The drawing under review shows one solid part. Ordinate dimensions are in mm from its lowest x, y, z. Coordinates: 2 decimals unless noted, no trailing zeros. Loops run counter-clockwise (first coordinate to the right, second up) from the corner with the lowest first, then second, coordinate; pieces in that order, holes last.
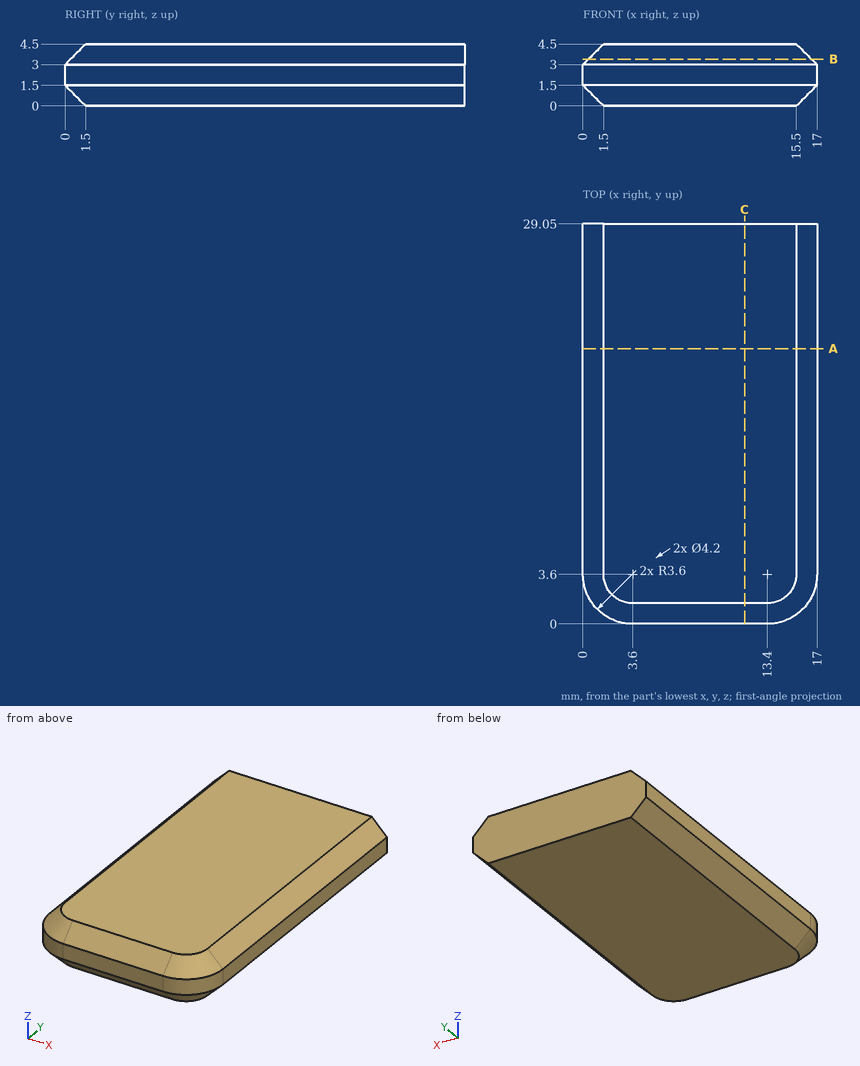
Q1. Take a section at B-B, the plane z = 3.4. Write out the cut boundary in (x, y), then the cut area to 3 significant figures.
Q2. Take a section at A-A, the plane y = 20. Write out the cut boundary in (x, z).
Q3. Take a section at C-C, the plane x = 11.75. Write out the cut boundary in (y, z).
Q4. For line 1 (Y direction, x = 12, z = 0.4); line 2 (Y direction, x = 6.75, z = 0.25); line 3 (Z direction, x = 16.25, y = 23.75), list the stretches that pass through material, from the lowest coordinate up.
Entries:
1. outline: (0.4, 3.6) arc R3.2 ccw to (3.6, 0.4) - (13.4, 0.4) arc R3.2 ccw to (16.6, 3.6) - (16.6, 29.05) - (0.4, 29.05) - close
1. area: 460 mm2
2. outline: (0, 1.5) - (1.5, 0) - (15.5, 0) - (17, 1.5) - (17, 3) - (15.5, 4.5) - (1.5, 4.5) - (0, 3) - close
3. outline: (0, 1.5) - (1.5, 0) - (29.05, 0) - (29.05, 4.5) - (1.5, 4.5) - (0, 3) - close
4. line 1: y = 1.1 to 29.05
4. line 2: y = 1.25 to 29.05
4. line 3: z = 0.75 to 3.75
